CAD build for the part. Positions are in the model's coordinates, mm. A direction names the side the tool comes from. Coordinates: 2 decimals unless noted, no trailing zeros. Loops run counter-clockwise (first coordinate to the right, second up) from the corner with the lowest first, then second, coordinate; pieces in that order, holes last. Notation, with made-up numbers: (32, 51.5) -> (84, 51.5) arc R27 ccw to (84, 80.5) -> close; hole circle Ø3 at (8, 80). An arc over 180 degrees is marked (long way). Write each question's results on one line, items separated by ' | '.
```python
from build123d import *

# Parameters (mm, degrees)
F0_R     = 3.25
F0_R_2   = 12.5
F1_DEPTH = 6
F2_R     = 21.5
F2_R_2   = 18.5
F3_DEPTH = 12
F4_R     = 21.5
F4_R_2   = 18.5
F5_DEPTH = 12
F6_SIZE  = 0.5


with BuildPart() as f1:
    # F0 (on Front) → F1 (new body)
    with BuildSketch(Plane.XZ):
        with BuildLine():
            Line((22.5, -26.809513), (22.5, 26.809513))
            ThreePointArc((22.5, 26.809513), (-14.790199, 31.721444), (-35, 0))
            ThreePointArc((-35, 0), (-14.790199, -31.721444), (22.5, -26.809513))
        make_face()
        with Locations((0, -27.5)):
            Circle(F0_R, mode=Mode.SUBTRACT)
        Circle(F0_R_2, mode=Mode.SUBTRACT)
        with Locations((0, 27.5)):
            Circle(F0_R, mode=Mode.SUBTRACT)
    extrude(amount=F1_DEPTH)

    # F2 (on face) → F3 (join)
    with BuildSketch(Plane.XZ.offset(6)):
        Circle(F2_R)
        Circle(F2_R_2, mode=Mode.SUBTRACT)
    extrude(amount=F3_DEPTH)

    # F4 (on face) → F5 (join)
    with BuildSketch(Plane(origin=(0, 0, 0), x_dir=(-1, 0, 0), z_dir=(0, 1, 0))):
        Circle(F4_R)
        Circle(F4_R_2, mode=Mode.SUBTRACT)
    extrude(amount=F5_DEPTH)

    # F6
    f6_edges = [f1.edges().sort_by_distance(p)[0] for p in [
        (-3.25, -6, 27.5),
        (-3.25, 0, 27.5),
        (-3.25, -6, -27.5),
        (-3.25, 0, -27.5),
        (18.5, 12, 0),
        (21.5, 12, 0),
        (-21.5, -18, 0),
        (-18.5, -18, 0),
    ]]
    chamfer(f6_edges, length=F6_SIZE)


solid = f1.part
```
Q1. Cut at D-D on x = -30. Write the cut outline in (y, z), and give its area (3 significant figures).
Results are:
outline: (-6, -18.03) -> (0, -18.03) -> (0, 18.03) -> (-6, 18.03) -> close | area: 216 mm^2
Q2. Cut at A-A on y = 2. Write the cut outline in (x, z), and give its area (3 significant figures).
Results are:
outline: circle Ø43 at (0, 0); hole circle Ø37 at (0, 0) | area: 377 mm^2
Q3. Cut at C-C on x = -23.5. Write the cut outline in (y, z), and give its area (3 significant figures).
Results are:
outline: (-6, -25.94) -> (0, -25.94) -> (0, 25.94) -> (-6, 25.94) -> close | area: 311 mm^2
Q4. Which spindle directions (+Z, -Z, +X, -X, +Y, -Y) get a long thin tool onto all of the face, cutting with end or side? Do faces 1 (the flat face through (22.5, -3, 0)), 2 (the flat face through (12.1, 0, -3.9)). Say none if no direction does.
Results are:
face 1: +Z, -Z, +X, +Y, -Y | face 2: +Y
Q5. Cut at B-B on x = 0. Give the number of separate pieces and of enclosed holes in the cut face, and give its area (3 significant figures).
Results are:
separate pieces: 4 | enclosed holes: 0 | area: 334 mm^2
Q6. Wall check: L1, parallel to Z at x = 0, y = -3.3; L2, parallel to Z at x = 0, y = -14; L3, parallel to Z at x = 10, y = -0.75. Give the ranges that are in metal, low to high. Write a range as from..to.
Results are:
L1: -35..-30.75, -24.25..-12.5, 12.5..24.25, 30.75..35 | L2: -21.5..-18.5, 18.5..21.5 | L3: -33.54..-7.5, 7.5..33.54
Q7. Drop flat-ended pins along their axis: pin 1 (2 mm diameter, centred on x = -5, y = -8.5, fed in from -Z); pin 2 (1 mm diameter, centred on y = -4, z = -5, fed in from -X); pin 3 (10 mm diameter, centred on x = 5, z = 16.5, fed in from -Y); pin 4 (8 mm diameter, centred on x = 9, y = 9, fed in from -Z). Give the stop position or say it passes through.
Results are:
pin 1: z = -21.12 | pin 2: x = -34.71 | pin 3: y = -18 | pin 4: z = -20.91
Q8. Pull direction Z, two halves, no side cores. Call faces 3 (the cylindrical face through (-2.799, -11.67, 21.317)), 4 (the cylindrical face through (-0.705, -2.965, 24.327)), 5 (the flat face through (-16, -18, -11)): +Z half, -Z half, draft (parallel to the pull), parting line (faces both ways), or undercut.
Results are:
face 3: parting line | face 4: undercut | face 5: draft
